Here's how the part is built. I have some questions about the finished solid (model axes, mm). Face numbers are marked on the shaded views. A direction names the side the tool comes from. Coordinates: 2 decimals unless noted, no trailing zeros. Write each loop counter-clockwise with the first axis right and the second up, starting at its lowest first coordinate (ties: lowest second). Pieces come first, ordered by that corner, then holes.
Autodesk Inventor part; units mm, degrees
ref_plane "YZ Plane" through (0, 0, 0) normal (1, 0, 0) x (0, 1, 0)
ref_plane "XZ Plane" through (0, 0, 0) normal (0, 1, 0) x (-1, 0, 0)
ref_plane "XY Plane" through (0, 0, 0) normal (0, 0, 1) x (1, 0, 0)
sketch "Skizze1" plane through (0, 0, 0) normal (0, 0, 1) x (1, 0, 0)
  line L0 (0, 0) -> (-25, 0)
  line L1 (-25, 0) -> (-25, 35)
  line L2 (-25, 35) -> (0, 35)
  line L3 (0, 35) -> (0, 0)
  dimension "d0" = 25
  dimension "d1" = 35
extrude "Extrusion1" add sketch "Skizze1" along normal blind 40
sketch "Skizze2" plane through (0, 0, 40) normal (0, 0, 1) x (1, 0, 0)
  line L0 (0, 6.5) -> (-16, 6.5)
  line L1 (-16, 6.5) -> (-16, 28.5)
  line L2 (-16, 28.5) -> (0, 28.5)
  line L3 (0, 28.5) -> (0, 6.5)
  line L4 (-25, 0) -> (0, 0)
  line L5 (0, 35) -> (-25, 35)
  line L6 (0, 0) -> (0, 35)
  dimension "d4" = 22
  dimension "d5" = 35
  dimension "d6" = 6.5
  dimension "d7" = 16
extrude "Extrusion2" cut sketch "Skizze2" against normal blind 40
sketch "Skizze3" plane through (0, 0, 40) normal (1, 0, 0) x (0, 0, -1)
  line L0 (0, 6.5) -> (0, 28.5)
  line L1 (40, 28.5) -> (40, 6.5)
  line L2 (40, 6.5) -> (0, 6.5)
  line L3 (40, 35) -> (0, 35)
  line L4 (40, 0) -> (0, 0)
  point P0 (20, 10)
  point P1 (20, 25)
  dimension "d10" = 15
  dimension "d11" = 20
  dimension "d12" = 40
  dimension "d15" = 35
  dimension "d16" = 10
hole "Bohrung1" at (0, 10, 20) at (0, 25, 20) direction (-1, 0, 0) diameter 5.5 end through all counterbore diameter 12.24 counterbore depth 16.5
sketch "Skizze4" plane through (-25, 35, 0) normal (0, 1, 0) x (1, 0, 0)
  line L0 (9, -40) -> (9, 0)
  line L1 (9, -40) -> (9, 0)
  line L2 (9, -13.88) -> (9, -26.12)
  line L3 (25, -40) -> (0, -40)
  line L4 (0, 0) -> (25, 0)
  point P0 (9, -14.9796)
  point P1 (9, -25.0204)
  point P2 (19, -5)
  point P3 (19, -35)
  dimension "d24" = 5
  dimension "d25" = 5
  dimension "d26" = 10
hole "Bohrung2" at (-6, 35, 5) at (-6, 35, 35) direction (0, -1, 0) diameter 3.4 end through all counterbore diameter 6.5 counterbore depth 2.4
sketch "Skizze5" plane through (-16, 28.5, 40) normal (0, -1, 0) x (1, 0, 0)
  circle A0 centre (10, -5) radius 2.25
  circle A1 centre (10, -5) radius 1.7
  point P0 (16, -40)
  dimension "d34" = 4.5
extrude "Extrusion3" add sketch "Skizze5" along normal blind 0.5
chamfer "Fase1" distance 0.3 angle 45 1 edges at (-8.25, 28.5, 35)
ref_plane "Arbeitsebene1" through (-25, 17.5, 0) normal (0, -1, 0) x (1, 0, 0)
ref_plane "Arbeitsebene2" through (0, 0, 20) normal (0, 0, 1) x (1, 0, 0)
mirror "Spiegeln1" about plane through (0, 0, 20) normal (0, 0, 1) of "Extrusion3", "Fase1"
mirror "Spiegeln2" about plane through (-25, 17.5, 0) normal (0, -1, 0) of "Extrusion3"
chamfer "Fase2" distance 0.3 angle 45 1 edges at (-8.25, 6.5, 35)
mirror "Spiegeln3" about plane through (0, 0, 20) normal (0, 0, 1) of "Extrusion3", "Spiegeln2", "Fase2"
fillet "Rundung1" radius 5.75 4 edges at (0, 3.25, 0) (0, 3.25, 40) (0, 31.75, 40) (0, 31.75, 0)
equation "\"d6\" = -0.5 * d4 + 0.5 * d5"
properties part number "belt_tensioner"
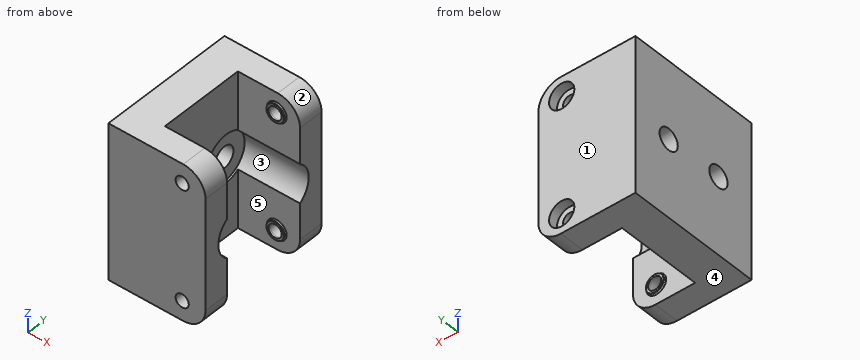
1) I need wall thicknesses on probe 1 along Z at (x, y) = (-6, 33.1); probe 2 along Y at (x, z) = (-21, 20); probe 3 along Z at (x, y) = (-6, 2.25). Which ranges of each line are inside material? Lowest first, please.
Values follow:
probe 1: z = 0 to 1.75, 8.25 to 31.75, 38.25 to 40
probe 2: y = 0 to 7.25, 12.75 to 22.25, 27.75 to 35
probe 3: z = 0 to 3.3, 6.7 to 33.3, 36.7 to 40
2) Imagine slicing it at D-D on y = 32. Please give me the cut outline in (x, z), then the cut area to 3 significant figures.
Values follow:
outline: (-25, 0) - (-5.75, 0) arc R5.75 ccw to (0, 5.75) - (0, 34.25) arc R5.75 ccw to (-5.75, 40) - (-25, 40) - close; hole circle Ø3.4 at (-6, 5); hole circle Ø3.4 at (-6, 35)
area: 968 mm2
3) On a 3-axis mill with a long thin cutter (end or side, diameter ignored), from which of +Z, -Z, +X, -X, +Y, -Y can I reach the whole of each face in a straight line? I mean the marked faces 4 and 5. Say none if no direction works.
Values follow:
face 4: -Z, +X, -X, +Y, -Y
face 5: none
4) Imagine slicing it at B-B on z = 20. Please give me the cut outline in (x, y).
Values follow:
outline: (-25, 0) - (0, 0) - (0, 3.88) - (-16.5, 3.88) - (-16.5, 7.25) - (-25, 7.25) - close; (-25, 12.75) - (-16.5, 12.75) - (-16.5, 16.12) - (-16, 16.12) - (-16, 18.88) - (-16.5, 18.88) - (-16.5, 22.25) - (-25, 22.25) - close; (-25, 27.75) - (-16.5, 27.75) - (-16.5, 31.12) - (0, 31.12) - (0, 35) - (-25, 35) - close
5) We'd pull the mould along Z, two halves only. Please class the marked faces 1, 2 and 3: pulls with the +Z half, pulls with the -Z half, needs draft (parallel to the pull), parting line crosses it, or undercut.
Values follow:
face 1: needs draft
face 2: pulls with the +Z half
face 3: undercut
6) Will these pins go through, and if not, where does the flat tip stop? pin 1 (10 mm diameter, centred on y = 22.5, z = 31.5, fed in from +X); pin 2 (5.5 mm diameter, centred on x = -6, z = 5, fed in from +Y).
Values follow:
pin 1: stops at x = -16
pin 2: stops at y = 32.6
7) Imagine slicing it at A-A on y = 10. Please give me the cut outline in (x, z), then the cut area to 3 significant figures.
Values follow:
outline: (-25, 0) - (-16, 0) - (-16, 13.88) - (-16.5, 13.88) - (-16.5, 17.25) - (-25, 17.25) - close; (-25, 22.75) - (-16.5, 22.75) - (-16.5, 26.12) - (-16, 26.12) - (-16, 40) - (-25, 40) - close
area: 307 mm2
8) Imagine slicing it at C-C on x = -10. Please give me the cut outline in (y, z).
Values follow:
outline: (0, 0) - (6.5, 0) - (6.5, 14.98) arc R6.12 cw to (6.5, 25.02) - (6.5, 40) - (0, 40) - close; (28.5, 0) - (35, 0) - (35, 40) - (28.5, 40) - (28.5, 25.02) arc R6.12 cw to (28.5, 14.98) - close
